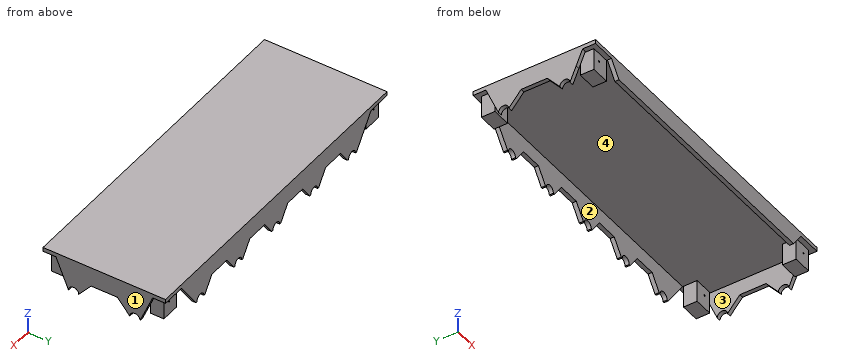
from build123d import *

# Parameters (mm, degrees)
F0_W      = 192.8
F0_H      = 71.8
F0_W_2    = 188
F0_H_2    = 67
F1_DEPTH  = 35
F2_R      = 3
F3_DEPTH  = 192.801
F4_R      = 3.9
F5_DEPTH  = 25
F6_R      = 3
F7_DEPTH  = 25
F8_W      = 192.8
F8_H      = 71.8
F8_W_2    = 188
F8_H_2    = 67
F11_DEPTH = 2.4
F12_DEPTH = 71.801
F13_DEPTH = 5
F14_START = -183.4
F14_DEPTH = 21.3
F15_W     = 11
F15_H     = 4.6784730554
F15_H_2   = 4.6253820807
F15_H_3   = 3.3215269446
F15_H_4   = 3.3746179193
F16_DEPTH = 13
F17_DEPTH = 25
F18_R     = 0.45
F19_DEPTH = 68.901


with BuildPart() as f1:
    # F0 (on Top) → F1 (new body)
    with BuildSketch(Plane.XY):
        Rectangle(F0_W, F0_H)
        Rectangle(F0_W_2, F0_H_2, mode=Mode.SUBTRACT)
    extrude(amount=F1_DEPTH)

    # F2 (on face) → F3 (cut, through all)
    with BuildSketch(Plane(origin=(-96.4, 0, 0), x_dir=(0, -1, 0), z_dir=(-1, 0, 0))):
        with Locations((-17.95, 17.5)):
            Circle(F2_R)
        with Locations((17.95, 17.5)):
            Circle(F2_R)
    extrude(amount=-F3_DEPTH, mode=Mode.SUBTRACT)

    # F4 (on face) → F5 (cut)
    with BuildSketch(Plane.XZ.offset(35.9)):
        with Locations((0, 17.5)):
            Circle(F4_R)
        with Locations((33, 17.5)):
            Circle(F4_R)
        with Locations((66, 17.5)):
            Circle(F4_R)
        with Locations((-33, 17.5)):
            Circle(F4_R)
        with Locations((-66, 17.5)):
            Circle(F4_R)
    extrude(amount=-F5_DEPTH, mode=Mode.SUBTRACT)

    # F6 (on face) → F7 (cut)
    with BuildSketch(Plane(origin=(0, 35.9, 0), x_dir=(-1, 0, 0), z_dir=(0, 1, 0))):
        with Locations((0, 17.5)):
            Circle(F6_R)
        with Locations((33, 17.5)):
            Circle(F6_R)
        with Locations((66, 17.5)):
            Circle(F6_R)
        with Locations((-33, 17.5)):
            Circle(F6_R)
        with Locations((-66, 17.5)):
            Circle(F6_R)
    extrude(amount=-F7_DEPTH, mode=Mode.SUBTRACT)

    # F8 (on face) → F11 (join)
    with BuildSketch(Plane.XY.offset(35)):
        Rectangle(F8_W, F8_H)
        Rectangle(F8_W_2, F8_H_2, mode=Mode.SUBTRACT)
        Rectangle(F8_W_2, F8_H_2)
    extrude(amount=F11_DEPTH)

    # F10 (on face) → F12 (cut, through all)
    with BuildSketch(Plane.XZ.offset(35.9)):
        with BuildLine():
            Line((-69.9, 17.5), (-76.02, 26))
            Line((-76.02, 26), (-94, 26))
            Line((-94, 26), (-94, 0))
            Line((-94, 0), (94, 0))
            Line((94, 0), (94, 26))
            Line((94, 26), (76.02, 26))
            Line((76.02, 26), (69.9, 17.5))
            ThreePointArc((69.9, 17.5), (66, 13.6), (62.1, 17.5))
            Line((62.1, 17.5), (55.98, 26))
            Line((55.98, 26), (43.02, 26))
            Line((43.02, 26), (36.9, 17.5))
            ThreePointArc((36.9, 17.5), (33, 13.6), (29.1, 17.5))
            Line((29.1, 17.5), (22.98, 26))
            Line((22.98, 26), (10.02, 26))
            Line((10.02, 26), (3.9, 17.5))
            ThreePointArc((3.9, 17.5), (0, 13.6), (-3.9, 17.5))
            Line((-3.9, 17.5), (-10.02, 26))
            Line((-10.02, 26), (-22.98, 26))
            Line((-22.98, 26), (-29.1, 17.5))
            ThreePointArc((-29.1, 17.5), (-33, 13.6), (-36.9, 17.5))
            Line((-36.9, 17.5), (-43.02, 26))
            Line((-43.02, 26), (-55.98, 26))
            Line((-55.98, 26), (-62.1, 17.5))
            ThreePointArc((-62.1, 17.5), (-66, 13.6), (-69.9, 17.5))
        make_face()
        Polygon((-76.02, 26), (-82.5, 35), (-94, 35), (-94, 26), align=None)
        Polygon((76.02, 26), (94, 26), (94, 35), (82.5, 35), align=None)
        with BuildLine():
            Line((-62.1, 17.5), (-69.9, 17.5))
            ThreePointArc((-69.9, 17.5), (-66, 13.6), (-62.1, 17.5))
        make_face()
        with BuildLine():
            Line((-29.1, 17.5), (-36.9, 17.5))
            ThreePointArc((-36.9, 17.5), (-33, 13.6), (-29.1, 17.5))
        make_face()
        with BuildLine():
            Line((3.9, 17.5), (-3.9, 17.5))
            ThreePointArc((-3.9, 17.5), (0, 13.6), (3.9, 17.5))
        make_face()
        with BuildLine():
            Line((36.9, 17.5), (29.1, 17.5))
            ThreePointArc((29.1, 17.5), (33, 13.6), (36.9, 17.5))
        make_face()
        with BuildLine():
            Line((69.9, 17.5), (62.1, 17.5))
            ThreePointArc((62.1, 17.5), (66, 13.6), (69.9, 17.5))
        make_face()
    extrude(amount=-F12_DEPTH, mode=Mode.SUBTRACT)

    # F9 (on face) → F13 (cut)
    with BuildSketch(Plane(origin=(-96.4, 0, 0), x_dir=(0, -1, 0), z_dir=(-1, 0, 0))):
        with BuildLine():
            Line((-20.95, 17.5), (-24.5562429894, 26))
            Line((-24.5562429894, 26), (-35.9, 26))
            Line((-35.9, 26), (-35.9, 0))
            Line((-35.9, 0), (35.9, 0))
            Line((35.9, 0), (35.9, 26))
            Line((35.9, 26), (24.5304559445, 26))
            Line((24.5304559445, 26), (20.95, 17.5))
            ThreePointArc((20.95, 17.5), (17.95, 14.5), (14.95, 17.5))
            Line((14.95, 17.5), (7.6885714286, 26))
            Line((7.6885714286, 26), (-7.6885714286, 26))
            Line((-7.6885714286, 26), (-14.95, 17.5))
            ThreePointArc((-14.95, 17.5), (-17.95, 14.5), (-20.95, 17.5))
        make_face()
        Polygon((-24.5562429894, 26), (-28.3746179193, 35), (-35.9, 35), (-35.9, 26), align=None)
        Polygon((35.9, 35), (28.3215269446, 35), (24.5304559445, 26), (35.9, 26), align=None)
    extrude(amount=-F13_DEPTH, mode=Mode.SUBTRACT)

    # F9 (on face) → F14 (cut)
    with BuildSketch(Plane(origin=(-96.4, 0, 0), x_dir=(0, -1, 0), z_dir=(-1, 0, 0)).offset(F14_START)):
        Polygon((-24.5562429894, 26), (-28.3746179193, 35), (-35.9, 35), (-35.9, 26), align=None)
        Polygon((35.9, 35), (28.3215269446, 35), (24.5304559445, 26), (35.9, 26), align=None)
        with BuildLine():
            Line((-20.95, 17.5), (-24.5562429894, 26))
            Line((-24.5562429894, 26), (-35.9, 26))
            Line((-35.9, 26), (-35.9, 0))
            Line((-35.9, 0), (35.9, 0))
            Line((35.9, 0), (35.9, 26))
            Line((35.9, 26), (24.5304559445, 26))
            Line((24.5304559445, 26), (20.95, 17.5))
            ThreePointArc((20.95, 17.5), (17.95, 14.5), (14.95, 17.5))
            Line((14.95, 17.5), (7.6885714286, 26))
            Line((7.6885714286, 26), (-7.6885714286, 26))
            Line((-7.6885714286, 26), (-14.95, 17.5))
            ThreePointArc((-14.95, 17.5), (-17.95, 14.5), (-20.95, 17.5))
        make_face()
    extrude(amount=-F14_DEPTH, mode=Mode.SUBTRACT)

    # F15 (on face) → F16 (join)
    with BuildSketch(Plane(origin=(0, 0, 35), x_dir=(1, 0, 0), z_dir=(0, 0, -1))):
        with Locations((-88, 30.6607634723)):
            Rectangle(F15_W, F15_H)
        with Locations((-88, -30.6873089597)):
            Rectangle(F15_W, F15_H_2)
        with Locations((88, -30.6873089597)):
            Rectangle(F15_W, F15_H_2)
        with Locations((88, 30.6607634723)):
            Rectangle(F15_W, F15_H)
        with Locations((88, 26.6607634723)):
            Rectangle(F15_W, F15_H_3)
        with Locations((88, -26.6873089597)):
            Rectangle(F15_W, F15_H_4)
        with Locations((-88, -26.6873089597)):
            Rectangle(F15_W, F15_H_4)
        with Locations((-88, 26.6607634723)):
            Rectangle(F15_W, F15_H_3)
    extrude(amount=F16_DEPTH)

    # F10 (on face) → F17 (cut)
    with BuildSketch(Plane.XZ.offset(35.9)):
        with BuildLine():
            Line((-55.98, 26), (-76.02, 26))
            Line((-76.02, 26), (-69.9, 17.5))
            ThreePointArc((-69.9, 17.5), (-66, 21.4), (-62.1, 17.5))
            Line((-62.1, 17.5), (-55.98, 26))
        make_face()
        with BuildLine():
            Line((-22.98, 26), (-43.02, 26))
            Line((-43.02, 26), (-36.9, 17.5))
            ThreePointArc((-36.9, 17.5), (-33, 21.4), (-29.1, 17.5))
            Line((-29.1, 17.5), (-22.98, 26))
        make_face()
        with BuildLine():
            Line((10.02, 26), (-10.02, 26))
            Line((-10.02, 26), (-3.9, 17.5))
            ThreePointArc((-3.9, 17.5), (0, 21.4), (3.9, 17.5))
            Line((3.9, 17.5), (10.02, 26))
        make_face()
        with BuildLine():
            Line((43.02, 26), (22.98, 26))
            Line((22.98, 26), (29.1, 17.5))
            ThreePointArc((29.1, 17.5), (33, 21.4), (36.9, 17.5))
            Line((36.9, 17.5), (43.02, 26))
        make_face()
        with BuildLine():
            Line((76.02, 26), (55.98, 26))
            Line((55.98, 26), (62.1, 17.5))
            ThreePointArc((62.1, 17.5), (66, 21.4), (69.9, 17.5))
            Line((69.9, 17.5), (76.02, 26))
        make_face()
    extrude(amount=-F17_DEPTH, mode=Mode.SUBTRACT)

    # F18 (on face) → F19 (cut, through all)
    with BuildSketch(Plane(origin=(0, 33, 0), x_dir=(-1, 0, 0), z_dir=(0, 1, 0))):
        with Locations((-89, 30)):
            Circle(F18_R)
        with Locations((89, 30)):
            Circle(F18_R)
    extrude(amount=-F19_DEPTH, mode=Mode.SUBTRACT)


solid = f1.part
The model under review builds one solid part; all positions refer to its coordinate system, in mm. Face numbers are marked on the shaded views. Give positions to 0.01 mm unless a question says otherwise; leave off trailing zeros. Loops run counter-clockwise (first coordinate to the right, second up) from the corner with the lowest first, then second, coordinate; pieces in that order, holes last. Notation, with made-up numbers: (-34, -35.5) -> (-21, -35.5) arc R31 ccw to (-21, -9.5) -> close; hole circle Ø5 at (-21, -15). An arc over 180 degrees is marked (long way). Answer as a JSON object with one key per item and string values. Group by question number.
Q1. Draft analysis for pull direction X (two halves, no side actions). For the marked faces 1, 2, 3 and 4, state which applies: pulls with the +X half, pulls with the -X half, needs draft (parallel to the pull), parting line crosses it, or undercut.
Q2. Wall thickness on line 1 along X through (y, z) = (-30, 30); line 2 along Y through (x, z) = (72, 27.5); line 3 along Z through (x, y) = (-89, -29): over which ranges is each line inside the solid? List them lowest first.
Q3. Take a section at A-A (y = -17.95). Write out the cut boundary in (x, z), plus the area to 3 significant figures.
Q4. Take a section at C-C (z = 32.25). State how many separate pieces and enclosed holes the cut face has, plus the area to 3 significant figures.
Q5. Take a section at B-B (x = -66). Write out the cut boundary in (y, z).
Q6. Insertion check: pin 1 (4 mm diameter, centred on x = 88.5, y = 27, fed in from -Z); pin 2 (2 mm diameter, centred on x = -61, y = -2.5, fed in from -Z); pin 3 (4 mm diameter, centred on y = 31, z = 30, fed in from -X). Each pin has a flat end and moves straight along its axis. Give the tip position at first contact, or say it passes through.
Answer below:
{
 "1": {"face 1": "pulls with the +X half", "face 2": "needs draft", "face 3": "undercut", "face 4": "undercut"},
 "2": {"line 1": "x = -93.5 to -89.45, -88.55 to -82.5, 82.5 to 88.55, 89.45 to 93.5", "line 2": "y = -35.9 to -33.5, 33.5 to 35.9", "line 3": "z = 22 to 29.55, 30.45 to 37.4"},
 "3": {"outline": "(-96.4, 20.5) -> (-94, 20.5) -> (-94, 35) -> (94, 35) -> (94, 20.5) -> (96.4, 20.5) -> (96.4, 37.4) -> (-96.4, 37.4) -> close", "area": "532 mm2"},
 "4": {"separate pieces": "8", "enclosed holes": "0", "area": "1,390 mm2"},
 "5": {"outline": "(-35.9, 26) -> (-33.5, 26) -> (-33.5, 35) -> (33.5, 35) -> (33.5, 20.5) -> (35.9, 20.5) -> (35.9, 37.4) -> (-35.9, 37.4) -> close"},
 "6": {"pin 1": "stops at z = 22", "pin 2": "stops at z = 35", "pin 3": "stops at x = -93.5"}
}
